Autodesk Inventor part; units mm, degrees
ref_plane "YZ Plane" through (0, 0, 0) normal (1, 0, 0) x (0, 1, 0)
ref_plane "XZ Plane" through (0, 0, 0) normal (0, 1, 0) x (-1, 0, 0)
ref_plane "XY Plane" through (0, 0, 0) normal (0, 0, 1) x (1, 0, 0)
sketch "Sketch1" plane through (0, 0, 0) normal (0, 0, 1) x (1, 0, 0)
  line L0 (18, 0) -> (18, 6.5785)
  line L1 (18, 6.5785) -> (9, 6.5785)
  line L2 (9, 6.5785) -> (9, 5.25)
  line L3 (7, 5.5) -> (-7, 5.5)
  line L4 (-7, 5.5) -> (-7, 0)
  line L5 (-7, 0) -> (18, 0)
  line L6 (7, 5.5) -> (7, 5.25)
  line L7 (7, 5.25) -> (9, 5.25)
  point P0 (0, 0)
  dimension "d0" = 25
  dimension "d1" = 18
  dimension "d2" = 11
  dimension "d3" = 10.5
  dimension "d4" = 9
  dimension "d5" = 2
  dimension "d13" = 13.157
revolve "Revolution1" add sketch "Sketch1" angle 360 about axis through (-7, 0, 0) along (1, 0, 0)
chamfer "Chamfer1" distance 1.5 angle 45 1 edges at (18, -6.5785, 0)
chamfer "Chamfer2" distance 0.5 angle 45 1 edges at (9, -6.5785, 0)
thread "Thread1"
sketch "Sketch2" plane through (0, 0, 0) normal (0, 0, 1) x (1, 0, 0)
  line L0 (0, 12) -> (-5, 12)
  line L1 (-5, 12) -> (-5, 6.5)
  line L2 (-5, 6.5) -> (-4.25, 6.5)
  line L3 (-4.25, 6.5) -> (-4.25, 0)
  line L4 (-4.25, 0) -> (0, 0)
  line L5 (0, 0) -> (0, 12)
  dimension "d16" = 12
  dimension "d17" = 10
  dimension "d18" = 8.5
  dimension "d19" = 5.5
revolve "Revolution2" add sketch "Sketch2" angle 360 about axis through (0, 0, 0) along (0, 1, 0)
chamfer "Chamfer3" distance 0.5 angle 45 3 edges at (5, 12, 0) (5, 6.5, 0) (-7, -5.5, 0)
sketch "Sketch3" plane through (0, 0, 0) normal (0, 0, 1) x (1, 0, 0)
  line L0 (18, 5.0785) -> (18, -5.0785)
  line L1 (18, 0) -> (18, 4.25)
  line L2 (18, 4.25) -> (8.0753, 2.5)
  line L3 (8.0753, 2.5) -> (8.0753, 0)
  line L4 (8.0753, 0) -> (18, 0)
  point P0 (0, 0)
  dimension "d24" = 8.5
  dimension "d25" = 10
  dimension "d26" = 5
revolve "Revolution3" cut sketch "Sketch3" angle 360 about axis through (8.0753, 0, 0) along (1, 0, 0)
sketch "Sketch4" plane through (18, 0, 0) normal (1, 0, 0) x (0, 0, -1)
  circle A0 centre (0, 0) radius 4.25
  point P0 (0, 0)
  point P1 (0, 0)
hole "Hole1" at (18, 0, 0) direction (-1, 0, 0) diameter 5 depth 20.5 tip angle 118
sketch "Sketch5" plane through (0, 12, 0) normal (0, 1, 0) x (1, 0, 0)
  circle A0 centre (0, 0) radius 4.5
hole "Hole2" at (0, 12, 0) direction (0, -1, 0) diameter 5 depth 14.5 tip angle 118
chamfer "Chamfer4" distance 0.5 angle 45 1 edges at (0, 12, -2.5)
sketch "Sketch6" plane through (0, 0, 0) normal (0, 0, 1) x (1, 0, 0)
  line L0 (-4.5, 12) -> (4.5, 12)
  line L1 (-1.75, 12) -> (1.75, 12)
  line L2 (1.75, 12) -> (1.75, 10)
  line L3 (1.75, 10) -> (-1.75, 10)
  line L4 (-1.75, 10) -> (-1.75, 12)
  point P0 (0, 0)
  point P1 (0, 10)
  dimension "d45" = 2
  dimension "d46" = 3.5
extrude "Extrusion1" cut sketch "Sketch6" along normal through all both and the other way through all
properties part number "Part020. Hydraulic elbow" material "Steel, Carbon"
Part model, mm, in its own coordinate system. A direction names the side the tool comes from. Round coordinates to 2 decimals unless told otherwise and drop trailing zeros. Loops run counter-clockwise (first coordinate to the right, second up) from the corner with the lowest first, then second, coordinate; pieces in that order, holes last.
Item 1: Drop flat-ended pins along their axis: P1, Ø2.5, axis at x = 2, z = 0.5, coming from the -Y side; P2, Ø1.6, axis at y = 10.5, z = 3.5, coming from the -X side; P3, Ø4, axis at x = 0, z = 0, coming from the +Y side. Give the stop position or say it passes through.
Item 2: Mould opens along Z. For faces 5 (the face through (-4.619, 9.218, 1.915)), 6 (the face through (0, -4, 0)), 7 (the face through (1.75, 11, -3)) say: +Z half, -Z half, draft (parallel to the pull), parting line (faces both ways), or undercut.
Item 3: Cut at A-A, the plane x = 7.5. Give the cut face in (y, z), then the cut area to 3 significant figures.
Item 4: 3-axis set-ups, long thin cutter, end or side, ignore diameter. For faces 1 (the face through (9, -5, -3)), 2 (the face through (-2.64, 11.64, -0.04)), 3 (the face through (1.75, 11, 3)), 4 (the face through (4.88, -2.48, 0.33)): which of +Z, -Z, +X, -X, +Y, -Y reach the whole face in a straight line?
Item 5: Drill centre lines: line 1 (Z direction, x = 4.25, y = 0); line 2 (Z direction, x = 0, y = 8); line 3 (X direction, y = -5.25, z = 0.75). Where is each one in solid material? Low to high.
Item 6: Cut at B-B, the plane x = 10.5. Give the cut face in (y, z).
A:
1. P1: stops at y = -5.5
1. P2: stops at x = -4.21
1. P3: stops at y = -2.8
2. face 5: parting line
2. face 6: undercut
2. face 7: draft
3. outline: circle Ø10.5 at (0, 0); hole circle Ø5 at (0, 0)
3. area: 67.0 mm2
4. face 1: none
4. face 2: +Y
4. face 3: +Z, -Z, +Y
4. face 4: +X
5. line 1: z = -5.5 to -2.5, 2.5 to 5.5
5. line 2: z = -5 to -2.5, 2.5 to 5
5. line 3: x = -6.7 to 7, 9 to 17.78
6. outline: circle Ø13.16 at (0, 0); hole circle Ø5.86 at (0, 0)
